The listing builds one solid part. Answer for the finished solid, in the listing's coordinates (mm). A direction names the side the tool comes from. Coordinates: 2 decimals unless noted, no trailing zeros. Order: outer loops, then holes, each group sorted by start corner. A loop starts at its lowest first (then second) coordinate and runs counter-clockwise, first axis right, second up.
from build123d import *

# Parameters (mm, degrees)
SKETCH1_W           = 53.4
SKETCH1_H           = 21
BOSS_EXTRUDE2_DEPTH = 6.33000004
SKETCH3_W           = 40.6
SKETCH3_H           = 19.8
CUT_EXTRUDE1_DEPTH  = 30.380416956
SKETCH4_W           = 3
SKETCH4_H           = 1.16
CUT_EXTRUDE2_DEPTH  = 55.789405002
SKETCH5_R           = 2
CUT_EXTRUDE3_DEPTH  = 6.33


with BuildPart() as part:
    # Sketch1 → Boss-Extrude2 (new body)
    with BuildSketch(Plane.XY):
        Rectangle(SKETCH1_W, SKETCH1_H)
    extrude(amount=BOSS_EXTRUDE2_DEPTH)

    # Sketch3 → Cut-Extrude1 (cut, through all)
    with BuildSketch(Plane.XY.offset(6.33000004)):
        Rectangle(SKETCH3_W, SKETCH3_H)
    extrude(amount=-CUT_EXTRUDE1_DEPTH, mode=Mode.SUBTRACT)

    # Sketch4 → Cut-Extrude2 (cut, through all)
    with BuildSketch(Plane.ZY.offset(26.7)):
        with Locations((1.5, 0)):
            Rectangle(SKETCH4_W, SKETCH4_H)
    extrude(amount=-CUT_EXTRUDE2_DEPTH, mode=Mode.SUBTRACT)

    # Sketch5 → Cut-Extrude3 (cut)
    with BuildSketch(Plane.XY.offset(6.33000004)):
        with Locations((-23.95, 5.1)):
            Circle(SKETCH5_R)
        with Locations(Location((-23.95, -5.1, 0), (0, 0, 180))):
            Circle(SKETCH5_R)
        with Locations((23.95, -5.1)):
            Circle(SKETCH5_R)
        with Locations(Location((23.95, 5.1, 0), (0, 0, 180))):
            Circle(SKETCH5_R)
    extrude(amount=-CUT_EXTRUDE3_DEPTH, mode=Mode.SUBTRACT)


solid = part.part
(1) Find section A-A on z = 2. Determine the outline of the cut face in (x, y), then the cut area to 3 significant figures.
(2) Find the intervals of material crossed by probe 1 along Y at (x, z) = (23.95, 1.75); probe 2 along Y at (x, z) = (23.95, 4.5); probe 3 along X at (y, z) = (-7.25, 4.75), in increasing order.
(3) The mould has two halves that part along Y. Classify faces 4 (the cylindrical face through (-25.948, 5.188, 3.209)), 5 (the flat face through (-26.7, 0, 4)), 6 (the flat face through (0, 10.5, 3)), 7 (the flat face through (0, -10.5, 3)): pulls with the +Y half, pulls with the -Y half, needs draft (parallel to the pull), parting line crosses it, or undercut.
(4) Given pin 1 Ø0.6 at (x, y) = (23.5, 0) entering from -Z, flat-ended and moving along its own axis, determine where the tip first touches the part or whether it passes through.
(5) A tool of negligible diameter and unlimited length cuts with its end or side. For faces 1 (the flat face through (-0.1, -10.1, 6.33)), 2 (the flat face through (20.3, -0.1, 3.2)), 3 (the flat face through (-24, 0, 3)), from which of +Z, -Z, +X, -X, +Y, -Y can it reach the whole face along a straight path? Write none if from no direction.
(6) Find section C-C on x = 23.95. Determine the outline of the cut face in (y, z).
(7) Find section B-B on y = 1.25. Determine the outline of the cut face in (x, z).
(8) Find section D-D on y = -5.1. Determine the outline of the cut face in (x, z), then the cut area to 3 significant figures.
Resolved:
1. outline: (-26.7, -10.5) - (26.7, -10.5) - (26.7, -0.58) - (20.3, -0.58) - (20.3, -9.9) - (-20.3, -9.9) - (-20.3, -0.58) - (-26.7, -0.58) - close; (-26.7, 0.58) - (-20.3, 0.58) - (-20.3, 9.9) - (20.3, 9.9) - (20.3, 0.58) - (26.7, 0.58) - (26.7, 10.5) - (-26.7, 10.5) - close; hole circle Ø4 at (-23.95, -5.1); hole circle Ø4 at (-23.95, 5.1); hole circle Ø4 at (23.95, -5.1); hole circle Ø4 at (23.95, 5.1)
1. area: 252 mm2
2. probe 1: y = -10.5 to -7.1, -3.1 to -0.58, 0.58 to 3.1, 7.1 to 10.5
2. probe 2: y = -10.5 to -7.1, -3.1 to 3.1, 7.1 to 10.5
2. probe 3: x = -26.7 to -20.3, 20.3 to 26.7
3. face 4: undercut
3. face 5: needs draft
3. face 6: pulls with the +Y half
3. face 7: pulls with the -Y half
4. pin 1: stops at z = 3
5. face 1: +Z, +X, -X, +Y, -Y
5. face 2: +Z, -Z
5. face 3: -Z, +X, -X
6. outline: (-10.5, 0) - (-7.1, 0) - (-7.1, 6.33) - (-10.5, 6.33) - close; (-3.1, 0) - (-0.58, 0) - (-0.58, 3) - (0.58, 3) - (0.58, 0) - (3.1, 0) - (3.1, 6.33) - (-3.1, 6.33) - close; (7.1, 0) - (10.5, 0) - (10.5, 6.33) - (7.1, 6.33) - close
7. outline: (-26.7, 0) - (-20.3, 0) - (-20.3, 6.33) - (-26.7, 6.33) - close; (20.3, 0) - (26.7, 0) - (26.7, 6.33) - (20.3, 6.33) - close
8. outline: (-26.7, 0) - (-25.95, 0) - (-25.95, 6.33) - (-26.7, 6.33) - close; (-21.95, 0) - (-20.3, 0) - (-20.3, 6.33) - (-21.95, 6.33) - close; (20.3, 0) - (21.95, 0) - (21.95, 6.33) - (20.3, 6.33) - close; (25.95, 0) - (26.7, 0) - (26.7, 6.33) - (25.95, 6.33) - close
8. area: 30.4 mm2
